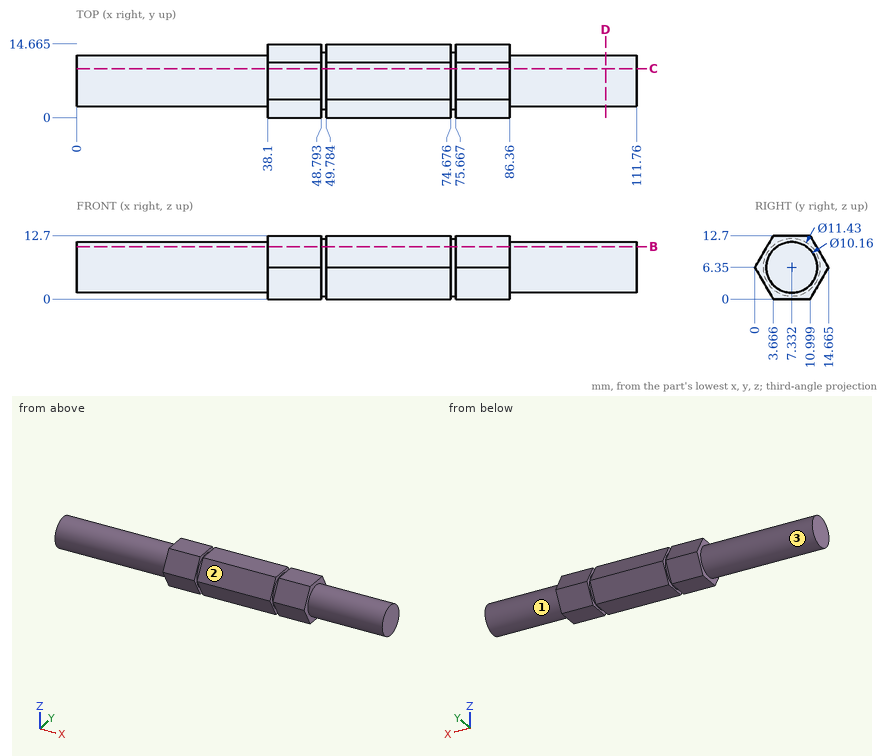
Input: dimensioned drawing with shaded views. Units: mm. Origin: part minimum x, y, z. A direction names the side the tool comes from. Round coordinates to 2 decimals unless told otherwise and drop trailing zeros. Order: outer loops, then holes, each group sorted by start corner. A loop starts at its lowest first (then second) coordinate and runs counter-clockwise, first axis right, second up. Notation, with made-up numbers: M 74.25,-35 L 127.25,-35 A26 ccw 127.25,-4 Z; hole C 61,31.25 d6. An arc over 180 degrees is marked long. Use one line per item in the form item = value. Start each with the question number.
Q1. Access query for the marked faces 1, 2 and 3. Directions: +Z, -Z, +X, -X, +Y, -Y. A direction counts if a zero-diameter tool reaches every point of the face in a straight line with its end or side. Return the directions, or none.
Q2. Cut plane D-D (x = 105.5). Return loops of the section in (y, z).
Q3. Material intervals for line 1 (X direction, y = 13.25, z = 6.5); line 2 (X direction, y = 4, z = 2); line 3 (Z direction, x = 74.5, y = 11) (1 decimal), sorted ascending. Write a range as [from, to].
Q4. Cut plane B-B (z = 10.5). Return loops of the section in (x, y).
Q5. Pin query (flat end, axial travel): pin 1 Ø6 at (x, y) = (94.5, 9.5) entering from +Z; pin 2 Ø1 at (x, y) = (71, 2) entering from -Z; pin 3 Ø6 at (x, z) = (12.5, 2) entering from -Y (1 decimal). Return the tip coordinate at first contact, or that it passes through.
Q6. Cut plane C-C (y = 9.75). Return loops of the section in (x, z), and give its area (3 significant figures).
Geometry results:
q1.face_1 = +X
q1.face_2 = +Z, +X, -X, -Y
q1.face_3 = -X
q2.outline = C 7.33,6.35 d10.16
q3.line_1 = [38.1, 48.79], [49.78, 74.68], [75.67, 86.36]
q3.line_2 = [38.1, 86.36]
q3.line_3 = [0, 12.7]
q4.outline = M 0,4.4 L 38.1,4.4 L 38.1,2.4 L 48.79,2.4 L 48.79,3.4 L 49.78,3.4 L 49.78,2.4 L 74.68,2.4 L 74.68,3.4 L 75.67,3.4 L 75.67,2.4 L 86.36,2.4 L 86.36,4.4 L 111.76,4.4 L 111.76,10.26 L 86.36,10.26 L 86.36,12.27 L 75.67,12.27 L 75.67,11.26 L 74.68,11.26 L 74.68,12.27 L 49.78,12.27 L 49.78,11.26 L 48.79,11.26 L 48.79,12.27 L 38.1,12.27 L 38.1,10.26 L 0,10.26 Z
q5.pin_1 = 11.43
q5.pin_2 = 2.02
q5.pin_3 = 2.4
q6.outline = M 0,1.88 L 38.1,1.88 L 38.1,0 L 48.79,0 L 48.79,1.17 L 49.78,1.17 L 49.78,0 L 74.68,0 L 74.68,1.17 L 75.67,1.17 L 75.67,0 L 86.36,0 L 86.36,1.88 L 111.76,1.88 L 111.76,10.82 L 86.36,10.82 L 86.36,12.7 L 75.67,12.7 L 75.67,11.53 L 74.68,11.53 L 74.68,12.7 L 49.78,12.7 L 49.78,11.53 L 48.79,11.53 L 48.79,12.7 L 38.1,12.7 L 38.1,10.82 L 0,10.82 Z
q6.area = 1,180 mm^2
